from build123d import *

# Parameters (mm, degrees)
EXTRUDE_1_DEPTH   = 2
HOLE_WIZARD_M81_D = 9
CHAMFER_1_SIZE    = 2


with BuildPart() as part:
    # Эскиз1 → Бобышка-Вытянуть1 (new body)
    with BuildSketch(Plane(origin=(0, 0, 0), x_dir=(1, 0, 0), z_dir=(0, 0, -1))):
        Polygon((0, 0), (0, 150), (150, 150), (150, 100), (100, 0), align=None)
    extrude(amount=EXTRUDE_1_DEPTH)

    # Отверстие с зазором M81 (through all)
    with Locations(Plane(origin=(0, 0, -2), x_dir=(1, 0, 0), z_dir=(0, 0, -1))):
        with Locations((75, 125), (25, 125), (25, 75), (25, 25), (125, 125), (75, 75), (75, 25)):
            Hole(HOLE_WIZARD_M81_D / 2)

    # Фаска1
    chamfer_1_edges = [part.edges().sort_by_distance(p)[0] for p in [
        (0, 0, -1),
        (0, -150, -1),
        (150, -150, -1),
    ]]
    chamfer(chamfer_1_edges, length=CHAMFER_1_SIZE)


solid = part.part
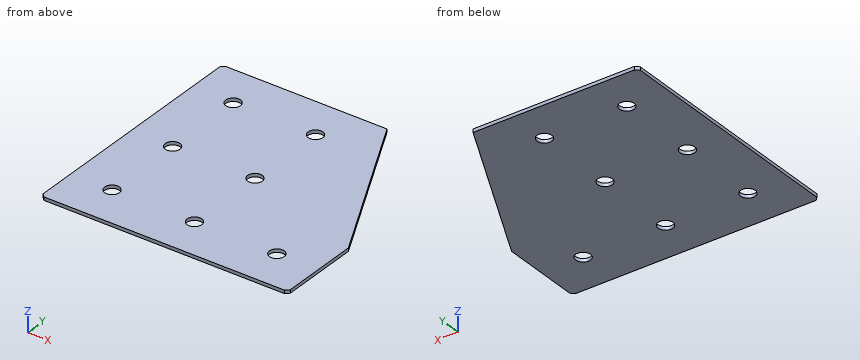
Part model, mm, in its own coordinate system. Coordinates: 2 decimals unless noted, no trailing zeros. Loops run counter-clockwise (first coordinate to the right, second up) from the corner with the lowest first, then second, coordinate; pieces in that order, holes last. Notation, with made-up numbers: (-13.75, 60) - (35.25, 60) arc R20 cw to (35.25, 79) - close; hole circle Ø11 at (-25, -33.75). An arc over 180 degrees is marked (long way). Write each question's results on one line, items separated by ' | '. Start each with the question number.
Q1. Slice it at B-B on y = -125. Give the cut face in (x, z), and give its area (3 significant figures).
Q2. Slice it at D-D on z = -0.85. Give the cut face in (x, y), and give its area (3 significant figures).
Q3. Probe line 1 along Y through (x, z) = (75, -0.5); line 2 along X through (y, z) = (-125, -1.15); line 3 along Y through (x, z) = (23, -0.65). List the from-to ranges inside material, lowest first.
Q4. Slice it at A-A on x = 125. Give the cut face in (y, z).
Q5. Slice it at C-C on x = 75. Give the cut face in (y, z), and give its area (3 significant figures).
Q6. Drop a flat-ended pin along its axis: pin 1 Ø7 at (x, y) = (25, -25) entering from -Z. Give the stop position or say it passes through.
Answer:
1) outline: (0, -2) - (20.5, -2) - (20.5, 0) - (0, 0) - close; (29.5, -2) - (70.5, -2) - (70.5, 0) - (29.5, 0) - close; (79.5, -2) - (120.5, -2) - (120.5, 0) - (79.5, 0) - close; (129.5, -2) - (150, -2) - (150, 0) - (129.5, 0) - close | area: 246 mm2
2) outline: (0, -148) - (2, -150) - (148, -150) - (150, -148) - (150, -100) - (100, 0) - (2, 0) - (0, -2) - close; hole circle Ø9 at (25, -125); hole circle Ø9 at (25, -75); hole circle Ø9 at (25, -25); hole circle Ø9 at (75, -125); hole circle Ø9 at (75, -75); hole circle Ø9 at (75, -25); hole circle Ø9 at (125, -125) | area: 19,500 mm2
3) line 1: y = -150 to -129.5, -120.5 to -79.5, -70.5 to -29.5, -20.5 to 0 | line 2: x = 0 to 20.5, 29.5 to 70.5, 79.5 to 120.5, 129.5 to 150 | line 3: y = -150 to -129.03, -120.97 to -79.03, -70.97 to -29.03, -20.97 to 0
4) outline: (-150, -2) - (-129.5, -2) - (-129.5, 0) - (-150, 0) - close; (-120.5, -2) - (-50, -2) - (-50, 0) - (-120.5, 0) - close
5) outline: (-150, -2) - (-129.5, -2) - (-129.5, 0) - (-150, 0) - close; (-120.5, -2) - (-79.5, -2) - (-79.5, 0) - (-120.5, 0) - close; (-70.5, -2) - (-29.5, -2) - (-29.5, 0) - (-70.5, 0) - close; (-20.5, -2) - (0, -2) - (0, 0) - (-20.5, 0) - close | area: 246 mm2
6) pin 1: passes through
